from build123d import *

# Parameters (mm, degrees)
CYLINDER032_R     = 2
CYLINDER032_DEPTH = 8
CYLINDER035_R     = 2
CYLINDER035_DEPTH = 8
CYLINDER038_R     = 1.6
CYLINDER038_DEPTH = 8
CYLINDER039_R     = 1.6
CYLINDER039_DEPTH = 8
CYLINDER037_W     = 7
CYLINDER037_H     = 8
CYLINDER037_ANGLE = 90
BOX025_W          = 78
BOX025_H          = 3
BOX025_DEPTH      = 7
BOX026_W          = 40
BOX026_H          = 3
BOX026_DEPTH      = 7
CYLINDER034_R     = 3.5
CYLINDER034_DEPTH = 8
CYLINDER031_R     = 3.5
CYLINDER031_DEPTH = 8
BOX027_W          = 40
BOX027_H          = 3
BOX027_DEPTH      = 7
CYLINDER036_W     = 7
CYLINDER036_H     = 8
CYLINDER036_ANGLE = 90


with BuildPart() as cuts:
    # Cylinder032 → Cylinder032 (new body)
    with BuildSketch(Plane(origin=(13.5, -2, 61.5), x_dir=(1, 0, 0), z_dir=(0, -1, 0))):
        Circle(CYLINDER032_R)
    extrude(amount=CYLINDER032_DEPTH)


with BuildPart() as cuts001:
    # Cylinder035 → Cylinder035 (new body)
    with BuildSketch(Plane(origin=(62.5, -2, 61.5), x_dir=(1, 0, 0), z_dir=(0, -1, 0))):
        Circle(CYLINDER035_R)
    extrude(amount=CYLINDER035_DEPTH)


with BuildPart() as m3screw:
    # Cylinder038 → Cylinder038 (new body)
    with BuildSketch(Plane(origin=(75.5, -2, 100.5), x_dir=(1, 0, 0), z_dir=(0, -1, 0))):
        Circle(CYLINDER038_R)
    extrude(amount=CYLINDER038_DEPTH)


with BuildPart() as c4oldcuts:
    # Cylinder039 → Cylinder039 (new body)
    with BuildSketch(Plane(origin=(2.5, -2, 100.5), x_dir=(1, 0, 0), z_dir=(0, -1, 0))):
        Circle(CYLINDER039_R)
    extrude(amount=CYLINDER039_DEPTH)

    # Fusion016: union cuts, cuts001, m3Screw
    add(cuts.part)
    add(cuts001.part)
    add(m3screw.part)


with BuildPart() as cylinder037:
    # Cylinder037 → Cylinder037 (revolve)
    with BuildSketch(Plane(origin=(0, -2, 98), x_dir=(1, 0, 0), z_dir=(0, 0, -1))):
        with Locations((3.5, 4)):
            Rectangle(CYLINDER037_W, CYLINDER037_H)
    revolve(axis=Axis((0, -2, 98), (0, -1, 0)), revolution_arc=CYLINDER037_ANGLE)


with BuildPart() as cube020:
    # Box025 → Box025 (new body)
    with BuildSketch(Plane(origin=(0, -5, 58), x_dir=(1, 0, 0), z_dir=(0, 0, 1))):
        with Locations((39, 1.5)):
            Rectangle(BOX025_W, BOX025_H)
    extrude(amount=BOX025_DEPTH)


with BuildPart() as cube021:
    # Box026 → Box026 (new body)
    with BuildSketch(Plane(origin=(7, -5, 58), x_dir=(0, 0, 1), z_dir=(-1, 0, 0))):
        with Locations((20, 1.5)):
            Rectangle(BOX026_W, BOX026_H)
    extrude(amount=BOX026_DEPTH)


with BuildPart() as cylinder034:
    # Cylinder034 → Cylinder034 (new body)
    with BuildSketch(Plane(origin=(62.5, -2, 61.5), x_dir=(1, 0, 0), z_dir=(0, -1, 0))):
        Circle(CYLINDER034_R)
    extrude(amount=CYLINDER034_DEPTH)


with BuildPart() as cylinder031:
    # Cylinder031 → Cylinder031 (new body)
    with BuildSketch(Plane(origin=(13.5, -2, 61.5), x_dir=(1, 0, 0), z_dir=(0, -1, 0))):
        Circle(CYLINDER031_R)
    extrude(amount=CYLINDER031_DEPTH)


with BuildPart() as fusion014:
    # Box027 → Box027 (new body)
    with BuildSketch(Plane(origin=(78, -5, 58), x_dir=(0, 0, 1), z_dir=(-1, 0, 0))):
        with Locations((20, 1.5)):
            Rectangle(BOX027_W, BOX027_H)
    extrude(amount=BOX027_DEPTH)

    # Fusion014: union Cube020, Cube021, Cylinder034, Cylinder031
    add(cube020.part)
    add(cube021.part)
    add(cylinder034.part)
    add(cylinder031.part)


with BuildPart() as c4hold001:
    # Cylinder036 → Cylinder036 (revolve)
    with BuildSketch(Plane(origin=(78, -2, 98), x_dir=(0, 0, 1), z_dir=(1, 0, 0))):
        with Locations((3.5, 4)):
            Rectangle(CYLINDER036_W, CYLINDER036_H)
    revolve(axis=Axis((78, -2, 98), (0, -1, 0)), revolution_arc=CYLINDER036_ANGLE)

    # Fusion015: union Cylinder037, Fusion014
    add(cylinder037.part)
    add(fusion014.part)

    # Cut024: cut c4oldCuts
    add(c4oldcuts.part, mode=Mode.SUBTRACT)


solid = c4hold001.part
The model under review builds one solid part; all positions refer to its coordinate system, in mm. A direction names the side the tool comes from. Give positions to 0.01 mm unless a question says otherwise; leave off trailing zeros. Order: outer loops, then holes, each group sorted by start corner. A loop starts at its lowest first (then second) coordinate and runs counter-clockwise, first axis right, second up. Notation, with made-up numbers: M -11.75,81.25 L -0.75,81.25 A30 cw -0.75,106.25 Z; hole C 36,56 d5. An arc over 180 degrees is marked long. Use one line per item in the form item = value. Start each with the question number.
Item 1: The part is to be moulded in two halves that separate along Z. For faces 4 (the flat face through (38, -3, 58)), 5 (the flat face through (38, -5, 61)), 6 (the cylindrical face through (13.24, -5.944, 63.483)), say which applies: pulls with the +Z half, pulls with the -Z half, needs draft (parallel to the pull), parting line crosses it, or undercut.
Item 2: For faces 1 (the flat face through (75, -8, 98)), 2 (the cylindrical face through (73.1, -6.1, 103)), 3 (the cylindrical face through (59.003, -7.465, 61.654)), list the 3-axis set-ups (+Z, -Z, +X, -X, +Y, -Y) from which the entire face can be reached by the end or side of a thin tool; tool diameter is ignored.
Item 3: We need section D-D on y = -3.5. Give the boundary of the cut face in (x, z).
Item 4: To check wall thickness, follow line 1 along X through (y, z) = (-4.5, 100.5); line 2 along Z through (x, y) = (62.5, -4); line 3 along X through (y, z) = (-3.75, 86.5). State the ranges of each line that lie inside material, in increasing order. Write a range as from..to.
Item 5: We need section A-A on y = -7.5. Give the boundary of the cut face in (x, z), plus the area to 3 significant figures.
Item 6: Insertion check: pin 1 Ø3.5 at (x, z) = (35, 63) entering from -Y; pin 2 Ø2.5 at (y, z) = (-4, 79) entering from -X; pin 3 Ø1.9 at (x, z) = (75.5, 100.5) entering from +Y; pin 4 Ø1.5 at (x, y) = (74.5, -7.5) entering from -Z. Each pin has a flat end and moves straight along its axis. Give the tip position at first contact, or say it passes through.
Item 7: We need section B-B on z = 61.5. Give the boundary of the cut face in (x, y).
Item 8: We need section C-C on x = 2.5. Give the boundary of the cut face in (y, z), plus the area to 3 significant figures.
Completed:
q1.face_4 = pulls with the -Z half
q1.face_5 = needs draft
q1.face_6 = undercut
q2.face_1 = -Z, +X, -X, -Y
q2.face_2 = +Z, +Y, -Y
q2.face_3 = -Y
q3.outline = M 0,58 L 78,58 L 78,105 A7 ccw 71,98 L 71,65 L 7,65 L 7,98 A7 ccw 0,105 Z; hole C 2.5,100.5 d3.2; hole C 13.5,61.5 d4; hole C 62.5,61.5 d4; hole C 75.5,100.5 d3.2
q4.line_1 = 0..0.9, 4.1..6.54, 71.46..73.9, 77.1..78
q4.line_2 = 58..59.5, 63.5..65
q4.line_3 = 0..7, 71..78
q5.outline = M 0,98 L 7,98 A7 ccw 0,105 Z; C 13.5,61.5 d7; C 62.5,61.5 d7; M 71,98 L 78,98 L 78,105 A7 ccw Z; hole C 2.5,100.5 d3.2; hole C 13.5,61.5 d4; hole C 62.5,61.5 d4; hole C 75.5,100.5 d3.2
q5.area = 113 mm²
q6.pin_1 = -5
q6.pin_2 = 0
q6.pin_3 = through
q6.pin_4 = 98
q7.outline = M 0,-5 L 10,-5 L 10,-10 L 11.5,-10 L 11.5,-2 L 0,-2 Z; M 15.5,-10 L 17,-10 L 17,-5 L 59,-5 L 59,-10 L 60.5,-10 L 60.5,-2 L 15.5,-2 Z; M 64.5,-10 L 66,-10 L 66,-5 L 78,-5 L 78,-2 L 64.5,-2 Z
q8.outline = M -10,98 L -5,98 L -5,58 L -2,58 L -2,98.9 L -10,98.9 Z; M -10,102.1 L -2,102.1 L -2,104.54 L -10,104.54 Z
q8.area = 147 mm²
